from build123d import *

# Parameters (mm, degrees)
SKETCH1_R           = 49.5
BOSS_EXTRUDE1_DEPTH = 5
CUT_EXTRUDE1_DEPTH  = 2
CUT_EXTRUDE2_DEPTH  = 2


with BuildPart() as part:
    # Sketch1 → Boss-Extrude1 (new body)
    with BuildSketch(Plane(origin=(0, 0, 0), x_dir=(1, 0, 0), z_dir=(0, 1, 0))):
        Circle(SKETCH1_R)
    extrude(amount=BOSS_EXTRUDE1_DEPTH)

    # Sketch2 → Cut-Extrude1 (cut)
    with BuildSketch(Plane(origin=(0, 5, 0), x_dir=(1, 0, 0), z_dir=(0, 1, 0))):
        with BuildLine():
            Line((14.5, 2), (0.364696883, 3.480947599))
            ThreePointArc((0.364696883, 3.480947599), (0, 3.5), (-0.364696883, 3.480947599))
            Line((-0.364696883, 3.480947599), (-14.5, 2))
            ThreePointArc((-14.5, 2), (-16.5, 0), (-14.5, -2))
            Line((-14.5, -2), (-3.185421861, -3.185421861))
            Line((-3.185421861, -3.185421861), (-2, -14.5))
            ThreePointArc((-2, -14.5), (0, -16.5), (2, -14.5))
            Line((2, -14.5), (3.185421861, -3.185421861))
            Line((3.185421861, -3.185421861), (14.5, -2))
            ThreePointArc((14.5, -2), (16.5, 0), (14.5, 2))
        make_face()
    extrude(amount=-CUT_EXTRUDE1_DEPTH, mode=Mode.SUBTRACT)

    # Sketch3 → Cut-Extrude2 (cut)
    with BuildSketch(Plane.XZ):
        with BuildLine():
            add(Edge.make_bspline(
                [(7.183697139, 7.183697139), (0, 87.002554241), (-7.183697139, 7.183697139)],
                knots=[1.862253121, 1.862253121, 1.862253121, 4.420932186, 4.420932186, 4.420932186], degree=2, weights=[1, 0.287347886, 1]))
            add(Edge.make_bspline(
                [(-7.183697139, 7.183697139), (-87.002554241, 0), (-7.183697139, -7.183697139)],
                knots=[5.003845775, 5.003845775, 5.003845775, 7.562524839, 7.562524839, 7.562524839], degree=2, weights=[1, 0.287347886, 1]))
            add(Edge.make_bspline(
                [(-7.183697139, -7.183697139), (0, -87.002554241), (7.183697139, -7.183697139)],
                knots=[5.003845775, 5.003845775, 5.003845775, 7.562524839, 7.562524839, 7.562524839], degree=2, weights=[1, 0.287347886, 1]))
            add(Edge.make_bspline(
                [(7.183697139, -7.183697139), (87.002554241, 0), (7.183697139, 7.183697139)],
                knots=[1.862253121, 1.862253121, 1.862253121, 4.420932186, 4.420932186, 4.420932186], degree=2, weights=[1, 0.287347886, 1]))
        make_face()
    extrude(amount=-CUT_EXTRUDE2_DEPTH, mode=Mode.SUBTRACT)


solid = part.part
Here's how the part is built. I have some questions about the finished solid (model axes, mm). Round coordinates to 2 decimals unless told otherwise and drop trailing zeros. Loops run counter-clockwise (first coordinate to the right, second up) from the corner with the lowest first, then second, coordinate; pieces in that order, holes last.
1. If we section it at C-C on x = -42: Write out the boundary of the cut face in (y, z), plus the area to 3 significant figures.
Answer list:
outline: (0, -26.2) - (5, -26.2) - (5, 26.2) - (0, 26.2) - close
area: 262 mm2
2. For P1, Ø2, axis at x = -5, y = 0.5, coming from the -Z side; P2, Ø2, axis at y = 2, z = 35.5, coming from the -X side, each with a flat end and sliding along its axis, tell me the tip position at first contact or that it passes through.
Answer list:
P1: stops at z = -49.34
P2: stops at x = -35.5
3. If we section it at A-A on y = 4: Write out the boundary of the cut face in (x, z), plus the area to 3 significant figures.
Answer list:
outline: circle Ø99 at (0, 0); hole (-14.5, -2) - (-0.36, -3.48) arc R3.5 ccw to (0.36, -3.48) - (14.5, -2) arc R2 ccw to (14.5, 2) - (3.19, 3.19) - (2, 14.5) arc R2 ccw to (-2, 14.5) - (-3.19, 3.19) - (-14.5, 2) arc R2 ccw to start
area: 7,460 mm2
4. If we section it at B-B on z = -30: Write out the boundary of the cut face in (x, y), plus the area to 3 significant figures.
Answer list:
outline: (-39.37, 0) - (39.37, 0) - (39.37, 5) - (-39.37, 5) - close
area: 394 mm2
5. We'd pull the mould along X, two halves only. Please class faces 1 (the face through (0, 3, 2)), 2 (the face through (-1, 5, -12)), 3 (the face through (-6.44, 2.46, -49.08)): +X half, -X half, draft (parallel to the pull), parting line (faces both ways), or undercut.
Answer list:
face 1: undercut
face 2: draft
face 3: parting line
6. If I drill on line 1 along X through (y, z) = (1.5, 19.5); line 2 along X through (y, z) = (1.35, -9.5); line 3 along Z through (x, y) = (-24, 0.55), over which ranges is the centre line in solid material (lowest first)?
Answer list:
line 1: x = -45.5 to -4.69, 4.69 to 45.5
line 2: x = -48.58 to -6.94, 6.94 to 48.58
line 3: z = -43.29 to -2.1, 2.1 to 43.29
